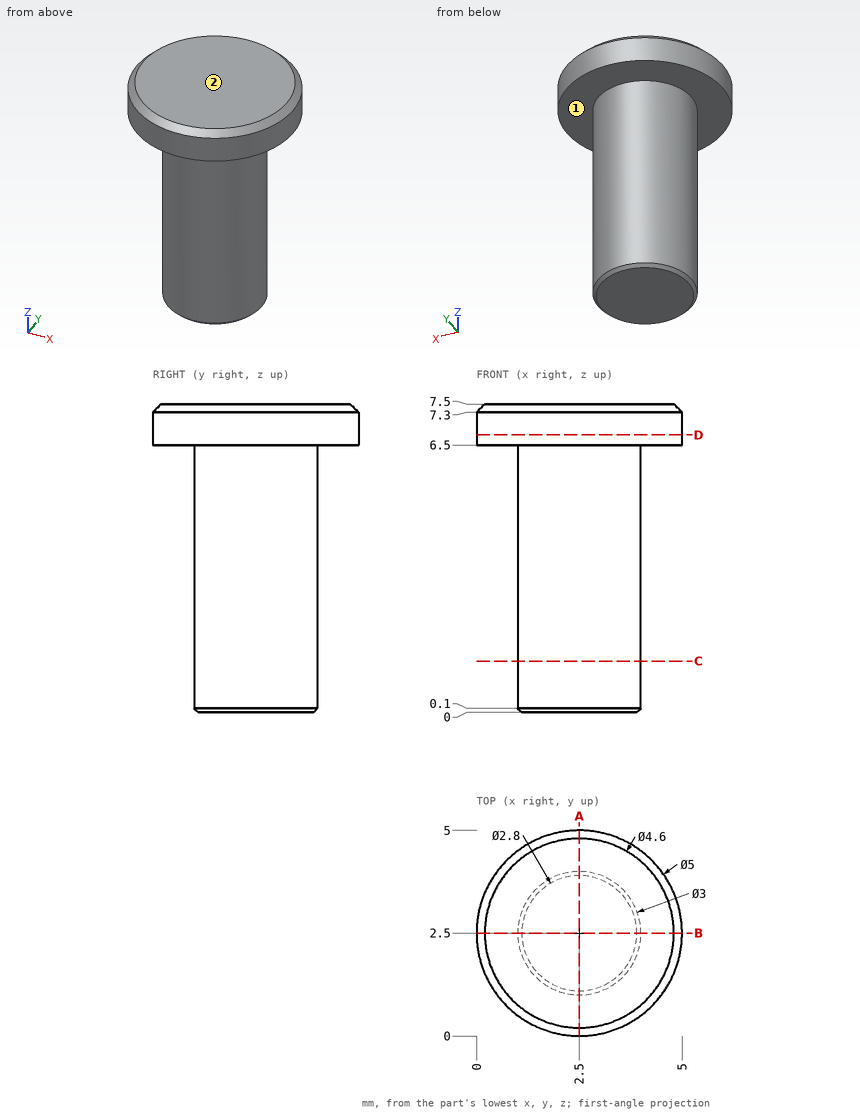
Can you work these out from the drawing? Everything is in mm from the part's minimum corner. A direction names the side the tool comes from. Give positions to 0.01 mm unless a question says otherwise; leave off trailing zeros. Loops run counter-clockwise (first coordinate to the right, second up) from the corner with the lowest first, then second, coordinate; pieces in that order, holes last. Notation, with made-up numbers: (22, 70.25) - (43, 70.25) arc R26 cw to (43, 103.25) - close; hole circle Ø6 at (22, -29.75). An arc over 180 degrees is marked (long way). Use one line per item in the form item = value.
1. I need wall thicknesses on probe 1 along Z at (x, y) = (4.55, 2.85); probe 2 along Y at (x, z) = (2.45, 6.25); probe 3 along Z at (x, y) = (4.75, 3.35). Which ranges of each line are inside material? Lowest first, please.
Response values:
probe_1 = 6.5 to 7.5
probe_2 = 1 to 4
probe_3 = 6.5 to 7.39
2. I'm going to push flat-ended pins straight in: pin 1 Ø1.5 at (y, z) = (3.5, 5.5) entering from +X; pin 2 Ø3 at (y, z) = (1.5, 4.5) entering from -X. Where does each tip first touch, or does it pass through?
Response values:
pin_1 = 3.98
pin_2 = 1
3. I want a section at A-A (x = 2.5). Please give me the cut outline in (y, z), and give its area (4 significant figures).
Response values:
outline = (0, 6.5) - (1, 6.5) - (1, 0.1) - (1.1, 0) - (3.9, 0) - (4, 0.1) - (4, 6.5) - (5, 6.5) - (5, 7.3) - (4.8, 7.5) - (0.2, 7.5) - (0, 7.3) - close
area = 24.45 mm²
4. I want a section at D-D (z = 6.75). Please give me the cut outline in (x, y), and give its area (3 significant figures).
Response values:
outline = circle Ø5 at (2.5, 2.5)
area = 19.6 mm²
5. I want a section at C-C (z = 1.25). Please give me the cut outline in (x, y).
Response values:
outline = circle Ø3 at (2.5, 2.5)
6. On a 3-axis mill with a long thin cutter (end or side, diameter ignored), from which of +Z, -Z, +X, -X, +Y, -Y can I reach the whole of each face in a straight line? I mean the marked faces 1 and 2. Say none if no direction works.
Response values:
face_1 = -Z
face_2 = +Z, +X, -X, +Y, -Y
